Can you work these out from the drawing? Everything is in mm from the part's minimum corner. A direction names the side the tool comes from. Coordinates: 2 decimals unless noted, no trailing zeros. Order: outer loops, then holes, each group sorted by start corner. A loop starts at its lowest first (then second) coordinate and runs counter-clockwise, first axis right, second up. Notation, with made-up numbers: (16.25, 7.25) -> (31.25, 7.25) arc R32 ccw to (31.25, 45.25) -> close; hole circle Ø4 at (48.5, 72.25). An arc over 180 degrees is marked (long way). Use a Markdown table: item, result. Add a question column.
1) If we section it at C-C (y = 5): Write out the boundary of the cut face in (x, z), plus the area to 3 significant figures.
2) If we section it at D-D (y = 2): Write out the boundary of the cut face in (x, z), plus the area to 3 significant figures.
3) Which directions (+Z, -Z, +X, -X, +Y, -Y) give clear straight access to the entire face, cutting with the end or side of a thin tool? Please do the marked faces 1, 2 and 3.
4) Thinking about a two-plate mould opening in X: for the marked faces 4, 5, 6 and 7, which applies, +X half, -X half, draft (parallel to the pull), parting line (faces both ways), or undercut?
5) If we section it at B-B (z = 6): Write out the boundary of the cut face in (x, y).
6) If we section it at A-A (x = 6): Write out the boundary of the cut face in (y, z), plus the area to 3 significant figures.
7) If I drill on L1, parallel to X at y = 0.85, z = 6; L2, parallel to Y at x = 18.4, z = 16; L3, parallel to X at y = 4, z = 14.5, over which ranges is the centre line in solid material (lowest first)? Write a range as [from, to].
8) Will these pins go through, and if not, where does the flat tip stop? pin 1 Ø0.8 at (x, y) = (6.5, 2) entering from -Z; pin 2 Ø1.5 at (x, y) = (13, 1) entering from +Z; pin 3 Ø4 at (x, z) = (6.5, 9.5) entering from +Y.
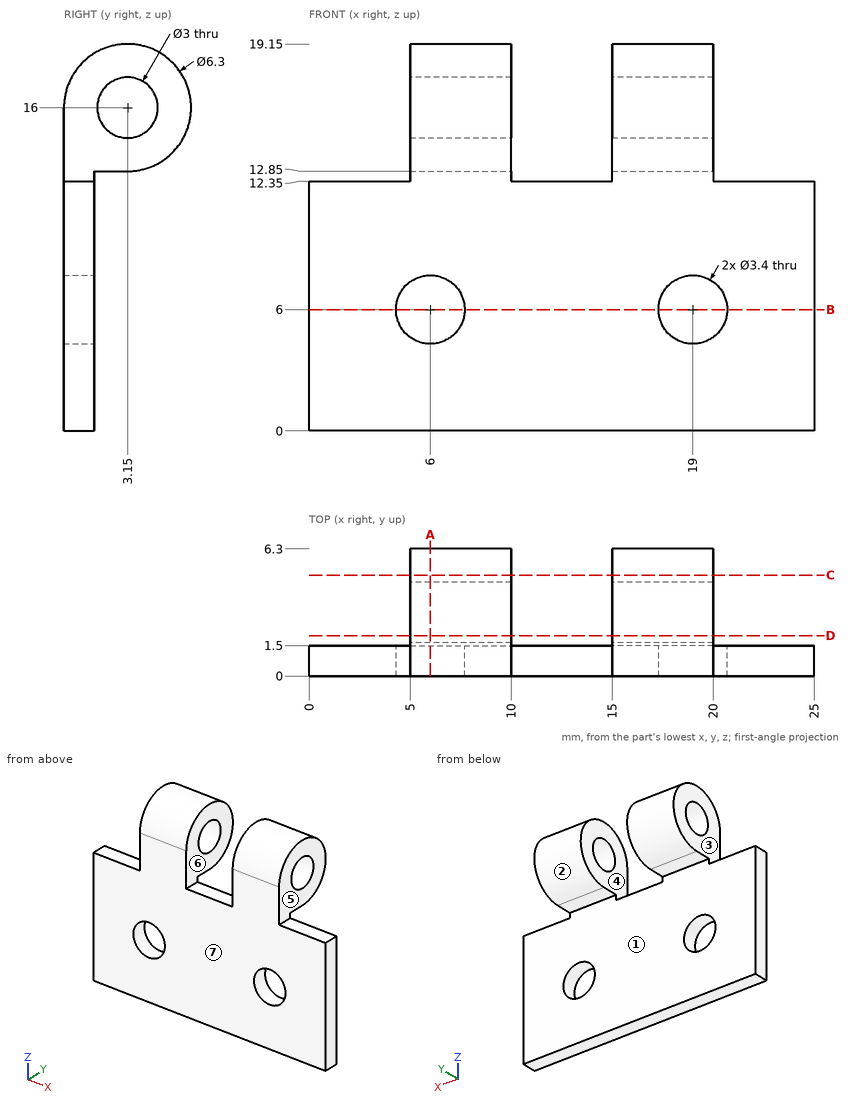
Answer sheet:
| question | item | result |
|---|---|---|
| 1 | outline | (5, 13.45) -> (10, 13.45) -> (10, 18.55) -> (5, 18.55) -> close; (15, 13.45) -> (20, 13.45) -> (20, 18.55) -> (15, 18.55) -> close |
| 1 | area | 51.0 mm2 |
| 2 | outline | (5, 12.85) -> (10, 12.85) -> (10, 15.04) -> (5, 15.04) -> close; (5, 16.96) -> (10, 16.96) -> (10, 18.93) -> (5, 18.93) -> close; (15, 12.85) -> (20, 12.85) -> (20, 15.04) -> (15, 15.04) -> close; (15, 16.96) -> (20, 16.96) -> (20, 18.93) -> (15, 18.93) -> close |
| 2 | area | 41.6 mm2 |
| 3 | face 1 | -Z, +X, -X, +Y |
| 3 | face 2 | +X, -X |
| 3 | face 3 | +Z, -X, +Y, -Y |
| 4 | face 4 | undercut |
| 4 | face 5 | +X half |
| 4 | face 6 | undercut |
| 4 | face 7 | draft |
| 5 | outline | (0, 0) -> (4.3, 0) -> (4.3, 1.5) -> (0, 1.5) -> close; (7.7, 0) -> (17.3, 0) -> (17.3, 1.5) -> (7.7, 1.5) -> close; (20.7, 0) -> (25, 0) -> (25, 1.5) -> (20.7, 1.5) -> close |
| 6 | outline | (0, 0) -> (1.5, 0) -> (1.5, 4.3) -> (0, 4.3) -> close; (0, 7.7) -> (1.5, 7.7) -> (1.5, 12.85) -> (3.15, 12.85) arc R3.15 ccw (long way) to (0, 16) -> close; hole circle Ø3 at (3.15, 16) |
| 6 | area | 40.4 mm2 |
| 7 | L1 | [0, 4.3], [7.7, 17.3], [20.7, 25] |
| 7 | L2 | [0, 1.65], [4.65, 6.3] |
| 7 | L3 | [5, 10], [15, 20] |
| 8 | pin 1 | z = 12.85 |
| 8 | pin 2 | z = 12.35 |
| 8 | pin 3 | y = 1.5 |
